Could you check a few things on this model? Use its own coordinates, in mm. A direction names the side the tool comes from. Coordinates: 2 decimals unless noted, no trailing zeros. Order: outer loops, then holes, each group sorted by start corner. A loop starts at its lowest first (then second) coordinate and runs counter-clockwise, first axis right, second up. Notation, with made-up numbers: (10.5, 7.5) - (24.5, 7.5) arc R18 cw to (24.5, 14.5) - close; hole circle Ø7 at (45.5, 70). An arc over 180 degrees is marked (long way). One line per item, written item: value.
from build123d import *

# Parameters (mm, degrees)
SKETCH1_W           = 90
SKETCH1_H           = 56
BOSS_EXTRUDE1_DEPTH = 4
SKETCH2_R           = 2.15
SKETCH2_R_2         = 1.7
CUT_EXTRUDE1_DEPTH  = 4
CUT_EXTRUDE2_DEPTH  = 2
BOSS_EXTRUDE3_DEPTH = 4
SKETCH6_R           = 9.5
CUT_EXTRUDE3_DEPTH  = 2
FILLET1_R           = 5
FILLET2_R           = 5


with BuildPart() as part:
    # Sketch1 → Boss-Extrude1 (new body)
    with BuildSketch(Plane(origin=(0, 0, 0), x_dir=(1, 0, 0), z_dir=(0, 1, 0))):
        Rectangle(SKETCH1_W, SKETCH1_H)
    extrude(amount=BOSS_EXTRUDE1_DEPTH)

    # Sketch2 → Cut-Extrude1 (cut)
    with BuildSketch(Plane(origin=(0, 4, 0), x_dir=(1, 0, 0), z_dir=(0, 1, 0))):
        with Locations(Location((-34.4, 0, 0), (0, 0, 270))):
            Circle(SKETCH2_R)
        with Locations(Location((34.4, 0, 0), (0, 0, 270))):
            Circle(SKETCH2_R)
        with Locations(Location((-39.002290859, -22, 0), (0, 0, 270))):
            Circle(SKETCH2_R_2)
        with Locations(Location((39, -22, 0), (0, 0, 270))):
            Circle(SKETCH2_R_2)
        with Locations(Location((39, 22, 0), (0, 0, 270))):
            Circle(SKETCH2_R_2)
        with Locations(Location((-39, 22, 0), (0, 0, 270))):
            Circle(SKETCH2_R_2)
    extrude(amount=-CUT_EXTRUDE1_DEPTH, mode=Mode.SUBTRACT)

    # Sketch3 → Cut-Extrude2 (cut)
    with BuildSketch(Plane.XZ):
        Polygon((30.825, -2.064027212), (34.4, -4.128054425), (37.975, -2.064027212), (37.975, 2.064027212), (34.4, 4.128054425), (30.825, 2.064027212), align=None)
        Polygon((-37.975, -2.064027212), (-34.4, -4.128054425), (-30.825, -2.064027212), (-30.825, 2.064027212), (-34.4, 4.128054425), (-37.975, 2.064027212), align=None)
    extrude(amount=-CUT_EXTRUDE2_DEPTH, mode=Mode.SUBTRACT)

    # Sketch4 → Boss-Extrude3 (add)
    with BuildSketch(Plane(origin=(0, 4, 0), x_dir=(1, 0, 0), z_dir=(0, 1, 0))):
        with BuildLine():
            Line((-45, -22), (-45, 22))
            ThreePointArc((-45, 22), (-67, 0), (-45, -22))
        make_face()
    extrude(amount=-BOSS_EXTRUDE3_DEPTH)

    # Sketch6 → Cut-Extrude3 (cut)
    with BuildSketch(Plane(origin=(0, 4, 0), x_dir=(1, 0, 0), z_dir=(0, 1, 0))):
        with Locations(Location((-54.5, 0, 0), (0, 0, 270))):
            Circle(SKETCH6_R)
    extrude(amount=-CUT_EXTRUDE3_DEPTH, mode=Mode.SUBTRACT)

    # Fillet1
    fillet1_edges = [part.edges().sort_by_distance(p)[0] for p in [
        (-45, 2, -28),
        (45, 2, -28),
        (45, 2, 28),
        (-45, 2, 28),
    ]]
    fillet(fillet1_edges, radius=FILLET1_R)

    # Fillet2
    fillet2_edges = [part.edges().sort_by_distance(p)[0] for p in [
        (-45, 2, -22),
        (-45, 2, 22),
    ]]
    fillet(fillet2_edges, radius=FILLET2_R)


solid = part.part
Item 1: I'm going to push flat-ended pins straight in: pin 1 Ø2 at (y, z) = (0.5, -0.5) entering from -X; pin 2 Ø3.5 at (x, z) = (-33.5, 0.5) entering from -Y; pin 3 Ø9.5 at (x, z) = (-56.5, 3.5) entering from +Y. Where does each tip first touch, or does it pass through?
Conclusion:
pin 1: x = -67
pin 2: y = 2
pin 3: y = 2
Item 2: I want a section at D-D on z = -13. Please give me the cut outline in (x, y).
Conclusion:
outline: (-62.75, 0) - (45, 0) - (45, 4) - (-62.75, 4) - close
Item 3: I want a section at C-C on z = 12.5. Please give me the cut outline in (x, y), then the cut area to 3 significant figures.
Conclusion:
outline: (-63.1, 0) - (45, 0) - (45, 4) - (-63.1, 4) - close
area: 432 mm²
Item 4: If I drill on probe 1 along X at (y, z) = (2.5, 0); probe 2 along X at (y, z) = (0.5, 23); probe 3 along Y at (x, z) = (-52, 1.5), over which ranges is the centre line in solid material (lowest first)?
Conclusion:
probe 1: -67 to -64, -45 to -36.55, -32.25 to 32.25, 36.55 to 45
probe 2: -45.9 to -40.38, -37.63 to 37.63, 40.37 to 45
probe 3: 0 to 2
Item 5: Thinking about a two-plate mould opening in X: for faces 1 (the face through (44, 2, -26)), 2 (the face through (-63.774, 3.014, -2.059)), 3 (the face through (-1, 2, -28)), which applies, pulls with the +X half, pulls with the -X half, needs draft (parallel to the pull), parting line crosses it, or undercut?
Conclusion:
face 1: pulls with the +X half
face 2: undercut
face 3: needs draft
Item 6: I want a section at A-A on z = 0. Please give me the cut outline in (x, y) (3 decimals), then the cut area to 3 significant figures.
Conclusion:
outline: (-67, 0) - (-37.975, 0) - (-37.975, 2) - (-36.55, 2) - (-36.55, 4) - (-45, 4) - (-45, 2) - (-64, 2) - (-64, 4) - (-67, 4) - close; (-32.25, 2) - (-30.825, 2) - (-30.825, 0) - (30.825, 0) - (30.825, 2) - (32.25, 2) - (32.25, 4) - (-32.25, 4) - close; (36.55, 2) - (37.975, 2) - (37.975, 0) - (45, 0) - (45, 4) - (36.55, 4) - close
area: 364 mm²
Item 7: I want a section at B-B on y = 0.7. Give the number of separate pieces and of enclosed holes in the cut face, then the cut area to 3 significant figures.
Conclusion:
separate pieces: 1
enclosed holes: 6
area: 5,660 mm²
Item 8: For faces 4 (the face through (-37.569, 2.028, 22.914)), 5 (the face through (-36.16, 0.99, 3.11)), 6 (the face through (-54, 2, 0)), which set-ups out of +Z, -Z, +X, -X, +Y, -Y let a thin tool reach every point of the face, with its end or its side?
Conclusion:
face 4: +Y, -Y
face 5: -Y
face 6: +Y
